Input: part model. Units: mm. Frame: model coordinates. A direction names the side the tool comes from. Coordinates: 2 decimals unless noted, no trailing zeros. Order: outer loops, then holes, each group sorted by start corner. A loop starts at its lowest first (then second) coordinate and runs counter-clockwise, first axis right, second up. Notation, with made-up numbers: (73, -32) -> (112, -32) arc R25 ccw to (112, -3) -> close; hole circle Ø6 at (-10.75, -33.5). An arc over 180 degrees is marked (long way). One line per item, written item: value. Start each with the question number.
from build123d import *

# Parameters (mm, degrees)
SKETCH_2_R           = 32.71124014
SKETCH_2_R_2         = 3.04999898
EXTRUDE_1_DEPTH      = 10
CUT_EXTRUDE_1_DEPTH  = 10
SKETCH_3_W           = 4.826
SKETCH_3_H           = 3.683
CUT_EXTRUDE_2_DEPTH  = 10
SKETCH_4_R           = 3.09999888
CUT_EXTRUDE_3_DEPTH  = 1.2
SKETCH_5_W           = 6.131993656
SKETCH_5_H           = 3.833791951
SKETCH_5_W_2         = 6.200437112
SKETCH_5_H_2         = 5.346426118
CUT_EXTRUDE_7_DEPTH  = 1.2
SKETCH_6_W           = 4.064
SKETCH_6_H           = 4.064
SKETCH_6_W_2         = 7.366
SKETCH_6_H_2         = 3.683
CUT_EXTRUDE_8_DEPTH  = 1.2
SKETCH_7_W           = 4.826
SKETCH_7_H           = 3.556
CUT_EXTRUDE_9_DEPTH  = 2.6
CHAMFER_1_SIZE       = 0.4
CUT_EXTRUDE_10_DEPTH = 1.7
SKETCH_9_W           = 5.344198096
SKETCH_9_H           = 4.530795449
CUT_EXTRUDE_11_DEPTH = 10
CHAMFER_3_SIZE       = 2
SKETCH_10_W          = 6.099936029
SKETCH_10_H          = 6.019169357
CUT_EXTRUDE_12_DEPTH = 10
CHAMFER_5_SIZE       = 1.1
CHAMFER_6_SIZE       = 2


with BuildPart() as part:
    # 草图2 → 凸台-拉伸1 (new body)
    with BuildSketch(Plane.XY):
        with Locations((99.695, 76.454)):
            Circle(SKETCH_2_R)
        with Locations((114.19499894, 101.56873768)):
            Circle(SKETCH_2_R_2, mode=Mode.SUBTRACT)
        with Locations((114.19511324, 51.33906674)):
            Circle(SKETCH_2_R_2, mode=Mode.SUBTRACT)
        with Locations((70.69477352, 76.454)):
            Circle(SKETCH_2_R_2, mode=Mode.SUBTRACT)
    extrude(amount=EXTRUDE_1_DEPTH)

    # 草图1 → 切除-拉伸1 (cut)
    with BuildSketch(Plane.XY):
        Polygon((72.39, 79.248), (74.422, 77.216), (74.422, 59.944), (78.359, 56.007), (81.788, 56.007), (83.312, 54.483), (86.614, 54.483), (87.757, 53.34), (88.519, 53.34), (89.662, 52.197), (89.662, 50.419), (91.059, 49.022), (107.061, 49.022), (107.315, 49.276), (107.315, 51.816), (122.809, 67.31), (122.809, 94.234), (121.158, 95.885), (106.172, 95.885), (103.886, 98.171), (103.886, 103.505), (103.378, 104.013), (89.408, 104.013), (89.281, 103.886), (89.281, 99.568), (88.265, 98.552), (84.61794354, 98.48969888), (82.677, 99.568), (80.137, 100.965), (80.01, 100.711), (78.61743992, 98.3237556), (77.22353618, 98.92855246), (69.52377256, 85.87810358), (69.596, 85.598), (69.596, 80.899), (70.866, 79.629), (71.501, 79.629), (71.882, 79.248), align=None)
    extrude(amount=CUT_EXTRUDE_1_DEPTH, mode=Mode.SUBTRACT)

    # 草图3 → 切除-拉伸2 (cut)
    with BuildSketch(Plane.XY):
        with Locations((72.009, 79.0575)):
            Rectangle(SKETCH_3_W, SKETCH_3_H)
    extrude(amount=CUT_EXTRUDE_2_DEPTH, mode=Mode.SUBTRACT)

    # 草图4 → 切除-拉伸3 (cut)
    with BuildSketch(Plane.XY):
        with Locations((128.69500042, 76.454)):
            Circle(SKETCH_4_R)
        with Locations((85.19500106, 51.3390007)):
            Circle(SKETCH_4_R)
        with Locations((85.19500106, 101.5689993)):
            Circle(SKETCH_4_R)
    extrude(amount=CUT_EXTRUDE_3_DEPTH, mode=Mode.SUBTRACT)

    # 草图5 → 切除-拉伸7 (cut)
    with BuildSketch(Plane.XY):
        with Locations((85.199003172, 99.987807393)):
            Rectangle(SKETCH_5_W, SKETCH_5_H)
        with Locations((85.195209049, 54.011411306)):
            Rectangle(SKETCH_5_W_2, SKETCH_5_H_2)
    extrude(amount=CUT_EXTRUDE_7_DEPTH, mode=Mode.SUBTRACT)

    # 草图6 → 切除-拉伸8 (cut)
    with BuildSketch(Plane.XY):
        Polygon((76.327, 58.293), (75.692, 58.293), (75.184, 58.293), (75.184, 56.388), (75.438, 56.134), (76.454, 56.134), (76.708, 55.88), (76.708, 54.483), (76.962, 54.229), (77.724, 54.229), (77.851, 54.102), (77.851, 53.594), (78.105, 53.34), (81.788, 53.34), (81.788, 58.293), align=None)
        with Locations((72.771, 65.278)):
            Rectangle(SKETCH_6_W, SKETCH_6_H)
        with Locations((127.635, 85.9155)):
            Rectangle(SKETCH_6_W_2, SKETCH_6_H_2)
        Polygon((94.742, 104.394), (94.742, 107.188), (103.886, 107.188), (103.886, 100.457), (94.742, 100.457), align=None)
    extrude(amount=CUT_EXTRUDE_8_DEPTH, mode=Mode.SUBTRACT)

    # 草图7 → 切除-拉伸9 (cut)
    with BuildSketch(Plane.XY):
        with Locations((91.694, 104.775)):
            Rectangle(SKETCH_7_W, SKETCH_7_H)
        Polygon((74.549, 67.945), (75.057, 67.945), (75.057, 70.612), (69.723, 70.612), (69.723, 67.945), align=None)
    extrude(amount=CUT_EXTRUDE_9_DEPTH, mode=Mode.SUBTRACT)

    # 倒角1
    chamfer_1_edges = [part.edges().sort_by_distance(p)[0] for p in [
        (69.300236993, 73.741480571, 10),
        (111.14499996, 101.56873768, 10),
        (111.14511426, 51.33906674, 10),
    ]]
    chamfer(chamfer_1_edges, length=CHAMFER_1_SIZE)

    # 草图8 → 切除-拉伸10 (cut)
    with BuildSketch(Plane.XY):
        Polygon((69.85, 68.072), (69.85, 72.39), (69.85, 73.536945765), (69.98685425, 73.673800015), (72.530800015, 73.673800015), (72.644, 73.787), (72.644, 78.994), (72.898, 79.248), (74.93, 79.248), (75.438, 78.74), (75.438, 72.898), (74.422, 71.882), (74.422, 68.072), align=None)
    extrude(amount=CUT_EXTRUDE_10_DEPTH, mode=Mode.SUBTRACT)

    # 草图9 → 切除-拉伸11 (cut)
    with BuildSketch(Plane.XY):
        with Locations((73.278206637, 75.553819753)):
            Rectangle(SKETCH_9_W, SKETCH_9_H)
    extrude(amount=CUT_EXTRUDE_11_DEPTH, mode=Mode.SUBTRACT)

    # 倒角3
    chamfer_3_edges = [part.edges().sort_by_distance(p)[0] for p in [
        (122.809, 80.772, 10),
        (121.9835, 95.0595, 10),
    ]]
    chamfer(chamfer_3_edges, length=CHAMFER_3_SIZE)

    # 草图10 → 切除-拉伸12 (cut)
    with BuildSketch(Plane.XY):
        with Locations((86.231031986, 100.876415322)):
            Rectangle(SKETCH_10_W, SKETCH_10_H)
    extrude(amount=CUT_EXTRUDE_12_DEPTH, mode=Mode.SUBTRACT)

    # 倒角5
    chamfer_5_edges = [part.edges().sort_by_distance(p)[0] for p in [
        (74.422, 66.616211014, 10),
    ]]
    chamfer(chamfer_5_edges, length=CHAMFER_5_SIZE)

    # 倒角6
    chamfer_6_edges = [part.edges().sort_by_distance(p)[0] for p in [
        (105.029, 97.028, 10),
    ]]
    chamfer(chamfer_6_edges, length=CHAMFER_6_SIZE)


solid = part.part
1) Section query B-B, the plane y = 66.5. Return the cut outline in (x, z).
2) Section query A-A, the plane y = 83. Return the cut outline in (x, z), plus the area to 3 significant figures.
3) Ray query, line 1 along X through (y, z) = (50, 3.5) (3 decimals); line 2 along Y through (x, z) = (115, 5) (3 decimals); line 3 along X through (y, z) = (52, 2.5). Return the intervals inside material, ascending. Write a range as from..to.
4) Mould query, pull axis X, two halves, no side actions, for faces 1 (the flat face through (124, 77, 0)), 2 (the flat face through (74.422, 67, 5)). Classes: +X half, -X half, draft (parallel to the pull), parting line (faces both ways), or undercut.
5) Access query for faces 3 (the conical face through (67.77, 75.26, 9.71)), 4 (the flat face through (86, 103.886, 5)), 5 (the flat face through (83, 103, 1.2)). Directions: +Z, -Z, +X, -X, +Y, -Y. A direction counts if a zero-diameter tool reaches every point of the face in a straight line with its end or side. Return the directions, or none.
6) Pin query (flat end, axial travel): pin 1 Ø2 at (y, z) = (60, 2.5) entering from -X; pin 2 Ø1.5 at (y, z) = (71.5, 1.5) entering from +X; pin 3 Ø5 at (x, z) = (74.5, 7.5) entering from +Y. Return the tip coordinate at first contact, or that it passes through.
7) Section query C-C, the plane x = 116.5. State how many separate pieces and enclosed holes the cut face has, plus the area to 3 significant figures.
Entries:
1. outline: (68.54, 0) -> (70.74, 0) -> (70.74, 1.2) -> (74.42, 1.2) -> (74.42, 8.9) -> (73.32, 10) -> (68.54, 10) -> close; (122, 0) -> (130.85, 0) -> (130.85, 10) -> (122, 10) -> close
2. outline: (67.65, 0) -> (69.6, 0) -> (69.6, 10) -> (67.65, 10) -> close; (122.81, 0) -> (131.74, 0) -> (131.74, 10) -> (124.81, 10) -> (122.81, 8) -> close
2. area: 107 mm2
3. line 1: x = 80.454..90.081, 107.315..111.455, 116.935..118.936
3. line 2: y = 47.544..48.397, 54.281..59.501, 95.885..98.627, 104.511..105.364
3. line 3: x = 77.97..89.66, 107.5..111.22, 117.17..121.42
4. face 1: draft
4. face 2: undercut
5. face 3: +Z
5. face 4: +Z, -Z
5. face 5: -Z
6. pin 1: stops at x = 70.86
6. pin 2: stops at x = 132.13
6. pin 3: stops at y = 100.01
7. separate pieces: 4
7. enclosed holes: 0
7. area: 132 mm2
